Here's the drawing with two shaded views (mm, measured from the low corner). I have some questions. Coordinates: 2 decimals unless noted, no trailing zeros. Write each loop counter-clockwise with the first axis right and the second up, starting at its lowest first coordinate (ties: lowest second). Pieces come first, ordered by that corner, then holes. Notation, with made-up numbers: (65, 59) -> (109, 59) arc R37 cw to (109, 97) -> close; hole circle Ø9 at (34.25, 67.25). An arc over 180 degrees is marked (long way). Put each result on its own line as item: value. Start each with the question number.
Item 1: I need wall thicknesses on line 1 (X direction, y = 25, z = 10.75) (1 decimal); line 2 (Y direction, x = 27, z = 12) (1 decimal); line 3 (Y direction, x = 25.5, z = 3.5) (1 decimal). Which ranges of each line are inside material? Lowest first, please. Write a range as [from, to].
Item 2: I want a section at A-A, the plane y = 19.5. List the corners of the cut face in (x, z) for me (1 decimal).
Item 3: If we mould it in two halves opening along X, with no side actions, what happens to the marked faces 1, 2 and 3? For each: released by +X, released by -X, zero draft, split by the parting line, or undercut.
Item 4: I want a section at B-B, the plane x = 34. List the corners of the cut face in (y, z) for me.
Item 5: For pin 1 (4 mm diameter, centred on y = 24, z = 6, fed in from +X); pin 2 (16 mm diameter, centred on x = 26.09, y = 25.55, fed in from +Z) (1 decimal); pin 3 (1.5 mm diameter, centred on x = 15.5, z = 4, fed in from -Y) (1 decimal); pin 4 (8 mm diameter, centred on x = 12.5, z = 2.5, fed in from -Y), each with a flat end and sliding along its axis, tell me the tip position at first contact or that it passes through.
Item 6: I want a section at D-D, the plane x = 40. List the corners of the cut face in (y, z) for me, then the cut area to 3 significant figures.
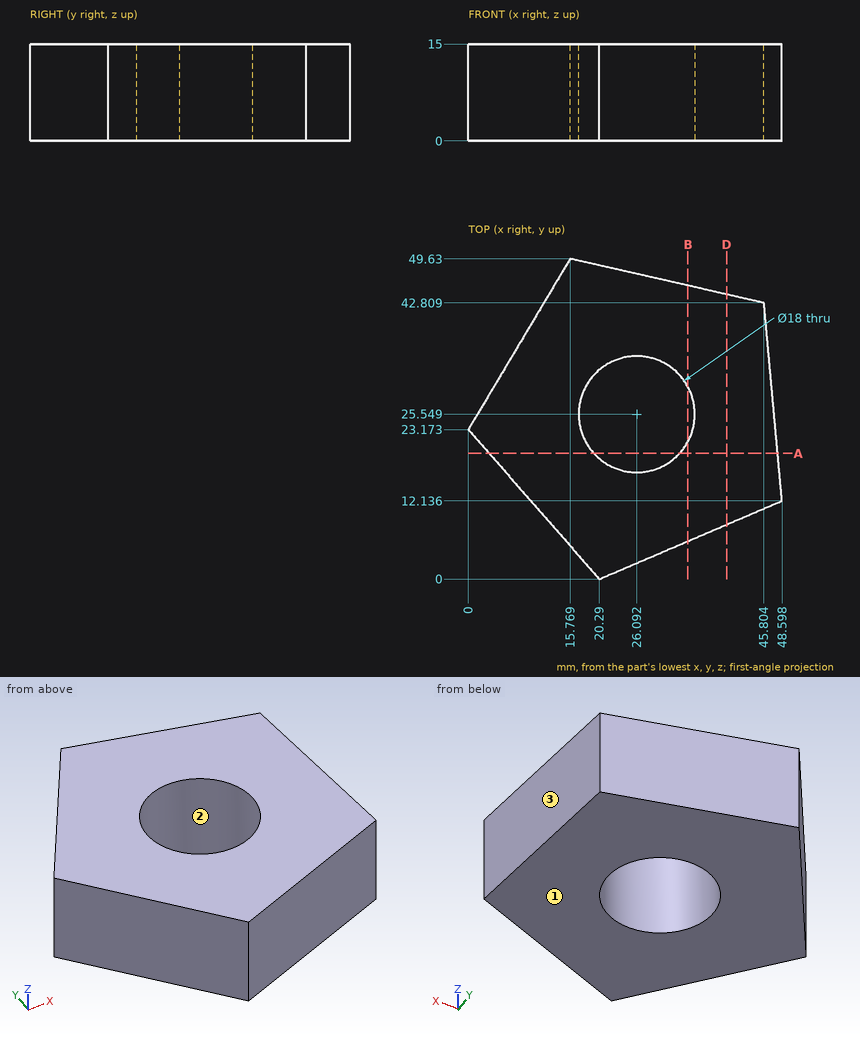
Calculated:
1. line 1: x = [1.1, 17.1], [35.1, 47.4]
1. line 2: y = [2.9, 16.6], [34.5, 47.1]
1. line 3: y = [2.2, 16.6], [34.5, 47.4]
2. outline: (3.2, 0) -> (19.4, 0) -> (19.4, 15) -> (3.2, 15) -> close; (32.8, 0) -> (47.9, 0) -> (47.9, 15) -> (32.8, 15) -> close
3. face 1: zero draft
3. face 2: undercut
3. face 3: released by +X
4. outline: (5.88, 0) -> (21.25, 0) -> (21.25, 15) -> (5.88, 15) -> close; (29.85, 0) -> (45.49, 0) -> (45.49, 15) -> (29.85, 15) -> close
5. pin 1: stops at x = 47.7
5. pin 2: passes through
5. pin 3: stops at y = 4.6
5. pin 4: stops at y = 4.33
6. outline: (8.45, 0) -> (44.13, 0) -> (44.13, 15) -> (8.45, 15) -> close
6. area: 535 mm2
